```python
from build123d import *

# Parameters (mm, degrees)
F0_W      = 31.75
F0_H      = 9.525
F1_DEPTH  = 3.175
F4_R      = 2.286
F8_R      = 2.286
F11_DEPTH = 9.525
F12_R     = 2


with BuildPart() as f1:
    # F0 (on Top) → F1 (new body)
    with BuildSketch(Plane.XY):
        with Locations((15.875, 4.7625)):
            Rectangle(F0_W, F0_H)
    extrude(amount=F1_DEPTH)

    # F5: sweep along a path in F3
    with BuildLine(Plane.YZ.offset(28.575)) as f5_path:
        Line((7.1374, 3.175), (7.1374, 9.525))
        Line((7.1374, 9.525), (11.6275280605, 14.0151280605))
    # F4 (on face) → F5 (sweep)
    with BuildSketch(Plane.XY.offset(3.175)):
        with Locations((28.575, 7.1374)):
            Circle(F4_R)
    sweep(path=f5_path.line, transition=Transition.RIGHT)

    # F9: sweep along a path in F7
    with BuildLine(Plane.YZ.offset(3.175)) as f9_path:
        Line((7.1374, 3.175), (7.1374, 9.525))
        Line((7.1374, 9.525), (11.6275280605, 14.0151280605))
    # F8 (on face) → F9 (sweep)
    with BuildSketch(Plane.XY.offset(3.175)):
        with Locations((3.175, 7.1374)):
            Circle(F8_R)
    sweep(path=f9_path.line, transition=Transition.RIGHT)

    # F10 (on face) → F11 (join, through all)
    with BuildSketch(Plane(origin=(0, 9.525, 0), x_dir=(-1, 0, 0), z_dir=(0, 1, 0))):
        with BuildLine():
            ThreePointArc((-27.2858537854, -10.9028537854), (-25.4, -6.35), (-23.5141462146, -10.9028537854))
            Line((-23.5141462146, -10.9028537854), (-22.7957257249, -11.6212742751))
            ThreePointArc((-22.7957257249, -11.6212742751), (-21.8362951849, -8.0872166969), (-24.4, -5.4723577049))
            Line((-24.4, -5.4723577049), (-24.4, 0))
            Line((-24.4, 0), (-26.4, 0))
            Line((-26.4, 0), (-26.4, -5.4723577049))
            ThreePointArc((-26.4, -5.4723577049), (-28.9637048151, -8.0872166969), (-28.0042742751, -11.6212742751))
            Line((-28.0042742751, -11.6212742751), (-27.2858537854, -10.9028537854))
        make_face()
        with BuildLine():
            Line((-5.35, 0), (-7.35, 0))
            Line((-7.35, 0), (-7.35, -5.4723577049))
            ThreePointArc((-7.35, -5.4723577049), (-9.9137048151, -8.0872166969), (-8.9542742751, -11.6212742751))
            Line((-8.9542742751, -11.6212742751), (-8.2358537854, -10.9028537854))
            ThreePointArc((-8.2358537854, -10.9028537854), (-6.35, -6.35), (-4.4641462146, -10.9028537854))
            Line((-4.4641462146, -10.9028537854), (-3.7457257249, -11.6212742751))
            ThreePointArc((-3.7457257249, -11.6212742751), (-2.7862951849, -8.0872166969), (-5.35, -5.4723577049))
            Line((-5.35, -5.4723577049), (-5.35, 0))
        make_face()
    extrude(amount=-F11_DEPTH)

    # F12
    f12_edges = [f1.edges().sort_by_distance(p)[0] for p in [
        (26.4, 4.7625, 0),
        (24.4, 4.7625, 0),
        (7.35, 4.7625, 0),
        (5.35, 4.7625, 0),
        (24.4, 4.7625, -5.472358),
        (26.4, 4.7625, -5.472358),
        (7.35, 4.7625, -5.472358),
        (5.35, 4.7625, -5.472358),
    ]]
    fillet(f12_edges, radius=F12_R)


solid = f1.part
```
Verification items for the finished model (mm, model axes). A direction names the side the tool comes from. Give positions to 0.01 mm unless a question says otherwise; leave off trailing zeros. Loops run counter-clockwise (first coordinate to the right, second up) from the corner with the lowest first, then second, coordinate; pieces in that order, holes last.
1. Section check A-A, the plane z = -3.75. Enter the section's corners in (x, y) (3 decimals), then the cut area to 3 significant figures.
2. Section check D-D, the plane x = 29.5. Enter the section's corners in (y, z) (3 decimals).
3. Thickness scan on line 1 (Y direction, x = 16.5, z = 1) (3 decimals); line 2 (Z direction, x = 25.4, y = 2.75) (3 decimals); line 3 (X direction, y = 12, z = 11.5). Record the ranges inside material, lowest first.
4. Set-up check for faces 4 (the flat face through (24.4, 5, -3)), 5 (the flat face through (15, 0, 1)), 6 (the cylindrical face through (4.75, 4.7, -0.57)), 7 (the cylindrical face through (2.7, 4.9, 6.1)), 8 (the cylindrical face through (26.645, 4.696, -5.15)): record each of +Z, -Z, +X, -X, +Y, -Y from which the full face is reachable in a straight line by a thin tool's end or side.
5. Section check B-B, the plane y = 4.5. Enter the section's corners in (x, z) (3 decimals), then the cut area to 3 significant figures.
6. Go/stop test with flat-tipped pins: pin 1 Ø2.5 at (y, z) = (5, -3.5) entering from -X; pin 2 Ø12 at (x, z) = (16.5, 4.5) entering from +Y (3 decimals); pin 3 Ø1.8 at (y, z) = (6, -3) entering from +X; pin 4 Ø4.5 at (x, z) = (6.35, -9.017) entering from +Y. Record where each tip stops, or that it passes through.
7. Mould release check, pull along Z, two halves, no side actions. Record for faces 1 (the flat face through (3.14, 11.6, 14.04)), 2 (the flat face through (30, 5, 0)), 3 (the flat face through (15, 9.525, 1)): released by +Z, released by -Z, zero draft, split by the parting line, or undercut.
8. Section check C-C, the plane x = 24. Enter the section's corners in (y, z) (3 decimals).
Geometry says:
1. outline: (5.35, 0) - (7.35, 0) - (7.35, 9.525) - (5.35, 9.525) - close; (24.4, 0) - (26.4, 0) - (26.4, 9.525) - (24.4, 9.525) - close
1. area: 38.1 mm2
2. outline: (0, 0) - (9.525, 0) - (9.525, 3.175) - (9.228, 3.175) - (9.228, 8.659) - (13.106, 12.537) - (10.149, 15.493) - (5.047, 10.391) - (5.047, 3.175) - (0, 3.175) - close
3. line 1: y = 0 to 9.525
3. line 2: z = -6.35 to 3.175
3. line 3: x = 2.15 to 4.2, 27.55 to 29.6
4. face 4: +Y, -Y
4. face 5: +Z, -Z, +X, -X, -Y
4. face 6: -X, +Y, -Y
4. face 7: none
4. face 8: +X, +Y, -Y
5. outline: (0, 0) - (3.35, 0) arc R2 cw to (5.35, -2) - (5.35, -4.19) arc R2 cw to (4.406, -5.889) arc R3.683 ccw to (3.746, -11.621) - (4.464, -10.903) arc R2.667 cw (long way) to (8.236, -10.903) - (8.954, -11.621) arc R3.683 ccw to (8.294, -5.889) arc R2 cw to (7.35, -4.19) - (7.35, -2) arc R2 cw to (9.35, 0) - (22.4, 0) arc R2 cw to (24.4, -2) - (24.4, -4.19) arc R2 cw to (23.456, -5.889) arc R3.683 ccw to (22.796, -11.621) - (23.514, -10.903) arc R2.667 cw (long way) to (27.286, -10.903) - (28.004, -11.621) arc R3.683 ccw to (27.344, -5.889) arc R2 cw to (26.4, -4.19) - (26.4, -2) arc R2 cw to (28.4, 0) - (31.75, 0) - (31.75, 3.175) - (0, 3.175) - close
5. area: 157 mm2
6. pin 1: stops at x = 5.27
6. pin 2: stops at y = 9.525
6. pin 3: stops at x = 26.4
6. pin 4: passes through
7. face 1: released by +Z
7. face 2: undercut
7. face 3: zero draft
8. outline: (0, -6.747) - (9.525, -6.747) - (9.525, -5.39) - (0, -5.39) - close; (0, -0.8) - (9.525, -0.8) - (9.525, 3.175) - (0, 3.175) - close
